Can you work these out from the model? Positions are in its coordinate system, mm. Face numbers are marked on the shaded views. A direction names the side the tool comes from. Round coordinates to 2 decimals unless told otherwise and drop trailing zeros. Loops run counter-clockwise (first coordinate to the right, second up) from the corner with the lowest first, then second, coordinate; pieces in that order, holes last. Notation, with made-up numbers: (-35, -21.75) -> (17, -21.75) arc R14 ccw to (17, 2.25) -> close; hole circle Ø4 at (45, -5.75). An arc over 180 degrees is marked (long way). Answer as a JSON object with one key per item and string values.
```python
from build123d import *

# Parameters (mm, degrees)
SKETCH2_R           = 5.969
BOSS_EXTRUDE1_DEPTH = 50.066
SKETCH7_R           = 2.5
CUT_EXTRUDE2_DEPTH  = 20


with BuildPart() as part:
    # Sketch1 → Revolve1 (revolve)
    with BuildSketch(Plane.XY, mode=Mode.PRIVATE) as revolve1_sk:
        Polygon((0, 0), (-10, 0), (0, 48.989794856), align=None)
    revolve(revolve1_sk.sketch.rotate(Axis((0, 48.989794856, 0), (0, -1, 0)), 90), axis=Axis((0, 48.989794856, 0), (0, -1, 0)))

    # Sketch2 → Boss-Extrude1 (add)
    with BuildSketch(Plane(origin=(0, 0, 0), x_dir=(1, 0, 0), z_dir=(0, 1, 0))):
        with Locations(Location((0, 0, 0), (0, 0, 90))):
            Circle(SKETCH2_R)
    extrude(amount=BOSS_EXTRUDE1_DEPTH)

    # Sketch7 → Cut-Extrude2 (cut)
    with BuildSketch(Plane.XZ):
        with Locations(Location((0, 0, 0), (0, 0, 270))):
            Circle(SKETCH7_R)
    extrude(amount=-CUT_EXTRUDE2_DEPTH, mode=Mode.SUBTRACT)


solid = part.part
```
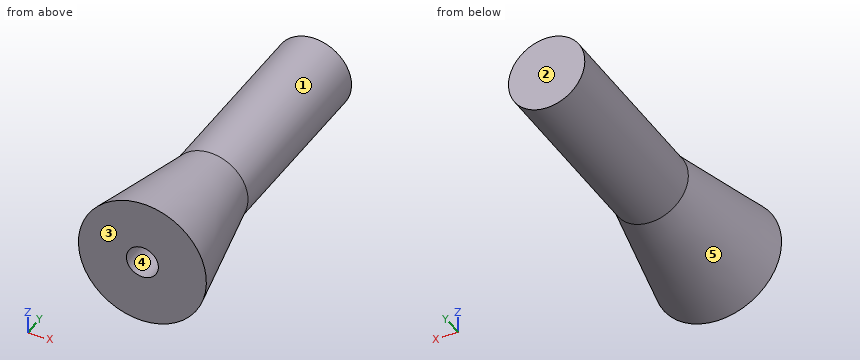
Q1. I want a section at A-A, the plane x = 0. Write out the boundary of the cut face in (y, z).
Determined:
{"outline": "(0, -10) -> (19.75, -5.97) -> (50.07, -5.97) -> (50.07, 5.97) -> (19.75, 5.97) -> (0, 10) -> (0, 2.5) -> (20, 2.5) -> (20, -2.5) -> (0, -2.5) -> close"}
Q2. I want a section at C-C, the plane y = 8.5. Write out the boundary of the cut face in (x, z).
Determined:
{"outline": "circle Ø16.53 at (0, 0); hole circle Ø5 at (0, 0)"}
Q3. We'd pull the mould along X, two halves only. Please class the marked faces 3, 4 and 5: pulls with the +X half, pulls with the -X half, needs draft (parallel to the pull), parting line crosses it, or undercut.
Determined:
{"face 3": "needs draft", "face 4": "undercut", "face 5": "parting line crosses it"}
Q4. I want a section at B-B, the plane z = 0. Write out the boundary of the cut face in (x, y).
Determined:
{"outline": "(-10, 0) -> (-2.5, 0) -> (-2.5, 20) -> (2.5, 20) -> (2.5, 0) -> (10, 0) -> (5.97, 19.75) -> (5.97, 50.07) -> (-5.97, 50.07) -> (-5.97, 19.75) -> close"}
Q5. I'm going to push flat-ended pins straight in: pin 1 (8 mm diameter, centred on x = -7, y = 35.5, fed in from -Z); pin 2 (6 mm diameter, centred on y = 16.5, z = 3, fed in from +X); pin 3 (1.5 mm diameter, centred on x = -0.5, z = -0.5, fed in from -Y); pin 4 (10 mm diameter, centred on x = -7, z = 1.5, fed in from +Y). Where does each tip first touch, or does it pass through?
Determined:
{"pin 1": "z = -5.16", "pin 2": "x = 7.02", "pin 3": "y = 20", "pin 4": "y = 50.07"}
Q6. If I drill on L1, parallel to Z at x = 1, y = 9; L2, parallel to Y at x = -1, z = 1.5; L3, parallel to Z at x = 7.75, y = 6.5, over which ranges is the centre line in solid material (lowest first)? Write a range as [from, to].
Determined:
{"L1": "[-8.1, -2.29], [2.29, 8.1]", "L2": "[20, 50.07]", "L3": "[-3.89, 3.89]"}
Q7. I want a section at D-D, the plane y = 29. Write out the boundary of the cut face in (x, z), then the cut area to 3 significant figures.
Determined:
{"outline": "circle Ø11.94 at (0, 0)", "area": "112 mm²"}
Q8. On a 3-axis mill with a long thin cutter (end or side, diameter ignored), from which of +Z, -Z, +X, -X, +Y, -Y can I reach the whole of each face in a straight line? I mean the marked faces 1 and 2. Say none if no direction works.
Determined:
{"face 1": "+Y", "face 2": "+Z, -Z, +X, -X, +Y"}
